Source: three-view drawing plus pictorial views. Frame: mm from the lowest corner of the part. A direction names the side the tool comes from. Coordinates: 2 decimals unless noted, no trailing zeros. Write each loop counter-clockwise with the first axis right and the second up, starting at its lowest first coordinate (ties: lowest second). Pieces come first, ordered by that corner, then holes. Notation, with made-up numbers: (14, -4) - (41, -4) arc R21 ccw to (41, 8) - close; hole circle Ø6 at (-18, 15.5). An arc over 180 degrees is marked (long way). Put each result on its own line as item: value.
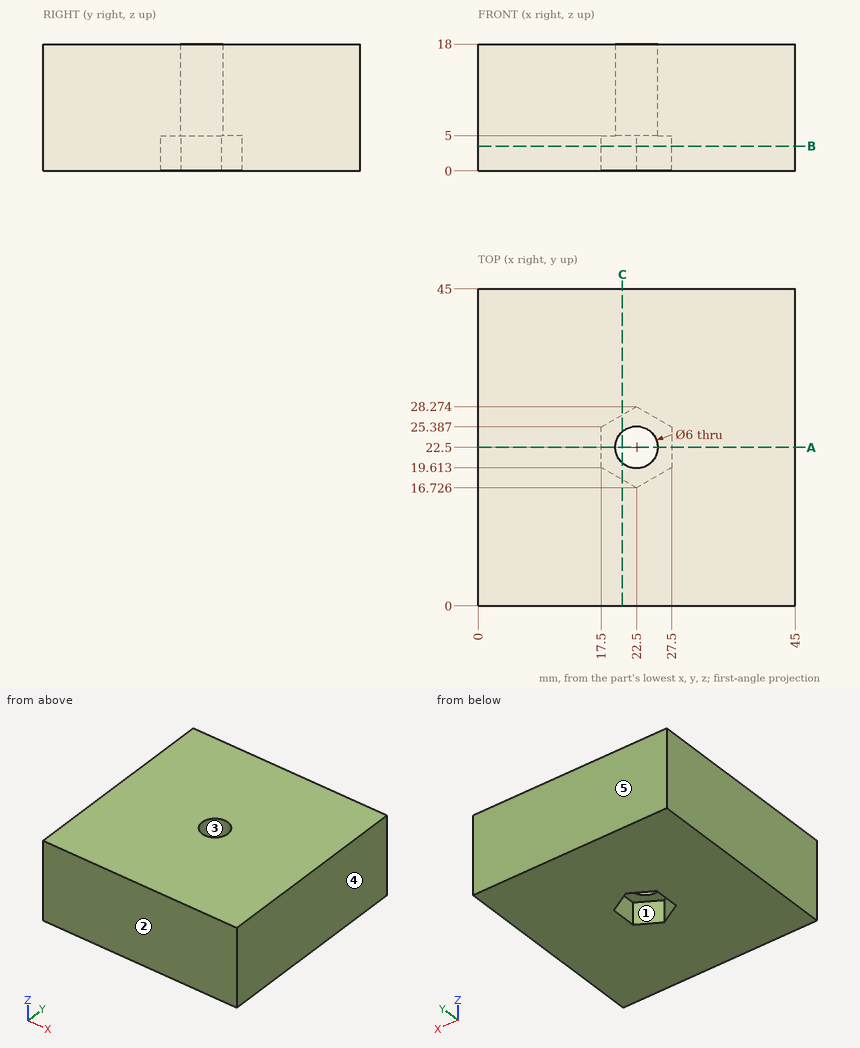
1. Section query C-C (x = 20.5). Return loops of the section in (y, z).
Answer below:
outline: (0, 0) - (17.88, 0) - (17.88, 5) - (20.26, 5) - (20.26, 18) - (0, 18) - close; (24.74, 5) - (27.12, 5) - (27.12, 0) - (45, 0) - (45, 18) - (24.74, 18) - close
2. Set-up query: the marked faces 1 and 2. Return all of +Z, -Z, +X, -X, +Y, -Y with unobstructed straight access to the full face (end or side cutting, diameter ignored); none if empty.
Answer below:
face 1: -Z
face 2: +Z, -Z, +X, -X, -Y
3. Section query B-B (z = 3.5). Return loops of the section in (x, y), then the cut area to 3 significant figures.
Answer below:
outline: (0, 0) - (45, 0) - (45, 45) - (0, 45) - close; hole (17.5, 19.61) - (22.5, 16.73) - (27.5, 19.61) - (27.5, 25.39) - (22.5, 28.27) - (17.5, 25.39) - close
area: 1,940 mm²
4. Pin query (flat end, axial travel): pin 1 Ø9.5 at (x, y) = (22.5, 22.5) entering from -Z. Return the tip coordinate at first contact, or that it passes through.
Answer below:
pin 1: stops at z = 5
5. Section query A-A (y = 22.5). Return loops of the section in (x, z), then the cut area to 3 significant figures.
Answer below:
outline: (0, 0) - (17.5, 0) - (17.5, 5) - (19.5, 5) - (19.5, 18) - (0, 18) - close; (25.5, 5) - (27.5, 5) - (27.5, 0) - (45, 0) - (45, 18) - (25.5, 18) - close
area: 682 mm²
6. Mould query, pull axis Y, two halves, no side actions, for the marked faces 3, 4 and 5. Classes: +Y half, -Y half, draft (parallel to the pull), parting line (faces both ways), or undercut.
Answer below:
face 3: undercut
face 4: draft
face 5: +Y half
7. Ray query, probe 1 along X at (y, z) = (22.5, 8.75); probe 2 along Y at (x, z) = (20.5, 13.75) (1 decimal). Return the intervals inside material, ascending. Write a range as from..to.
Answer below:
probe 1: x = 0..19.5, 25.5..45
probe 2: y = 0..20.3, 24.7..45
